Can you work these out from the model? Positions are in its coordinate system, mm. A direction names the side the tool comes from. Give positions to 0.01 mm unless a question says otherwise; leave off trailing zeros. Write each loop counter-clockwise with the first axis right and the second up, starting at its lowest first coordinate (ties: lowest second). Pieces come first, ordered by that corner, then holes. Notation, with made-up numbers: (-5, 43.5) - (39, 43.5) arc R13 ccw to (39, 52.5) - close; hole circle Ø8 at (89.25, -35.75). An arc over 180 degrees is marked (long way). Return JSON: item names as keys, results as strings. Group by question number.
from build123d import *

# Parameters (mm, degrees)
F2_R     = 10.5023561171
F3_DEPTH = 2.032
F4_R     = 1.2264204897
F6_R     = 8.280415088
F6_R_2   = 5.5395009723
F7_DEPTH = 5.334


# Not quite as in the source:
# - a fillet or chamfer that OpenCascade refuses, or shapes differently, is made with other operations: its cross-section is extruded or revolved along the edge and cut away or added


with BuildPart() as f1:
    # F0 (on Front) → F1 (revolve)
    with BuildSketch(Plane.XZ):
        with BuildLine():
            Line((0, 24.7002821416), (0, 0))
            Line((0, 0), (12.7, 0))
            ThreePointArc((12.7, 0), (15.1592770153, 1.3591062743), (12.7, 2.7182125486))
            ThreePointArc((12.7, 2.7182125486), (8.1323573281, 11.5574154189), (6.618256215, 21.3911514729))
            ThreePointArc((6.618256215, 21.3911514729), (7.1000680202, 23.0457168072), (6.618256215, 24.7002821416))
            Line((6.618256215, 24.7002821416), (0, 24.7002821416))
        make_face()
    revolve(axis=Axis((0, 0, 12.3501410708), (0, 0, -1)))

    # F2 (on face) → F3 (join)
    with BuildSketch(Plane.XY.offset(24.7002821416)):
        Circle(F2_R)
    extrude(amount=F3_DEPTH)

    # F4
    f4_edges = [f1.edges().sort_by_distance(p)[0] for p in [
        (-10.502356, 0, 26.732282),
    ]]
    fillet(f4_edges, radius=F4_R)

    # F5: fillet of radius 5.5188922036 on 1 edges, made by hand

    # F5_s1 → F5_t2 (revolve, cut)
    with BuildSketch(Plane.XZ):
        with BuildLine():
            ThreePointArc((10.5023561171, 25.5058616519), (9.1222760715, 24.9054922023), (7.631318916, 24.7002821416))
            Line((7.631318916, 24.7002821416), (7.631318916, 24.5899042975))
            Line((7.631318916, 24.5899042975), (10.5023561171, 24.5899042975))
            Line((10.5023561171, 24.5899042975), (10.6127339612, 24.7002821416))
            ThreePointArc((10.6127339612, 24.7002821416), (10.6127339612, 25.1030718967), (10.5597768612, 25.411595398))
            Line((10.5597768612, 25.411595398), (10.5023561171, 25.5058616519))
        make_face()
    revolve(axis=Axis((0, 0, 24.7002821416), (0, 0, 1)), mode=Mode.SUBTRACT)

    # F6 (on face) → F7 (join)
    with BuildSketch(Plane.XY.offset(26.7322821416)):
        Circle(F6_R)
        Circle(F6_R_2, mode=Mode.SUBTRACT)
    extrude(amount=F7_DEPTH)


solid = f1.part
1) Will these pins go through, and if not, where does the flat tip stop? pin 1 Ø8 at (x, y) = (11.5, 10.5) entering from +Z; pin 2 Ø1.5 at (x, y) = (0.5, -1) entering from +Z; pin 3 Ø3 at (y, z) = (-1.5, 22.5) entering from +X; pin 4 Ø1 at (x, z) = (-8.5, 13.5) entering from +Y.
2) I need wall thicknesses on line 1 along Y through (x, z) = (0, 30.35); line 2 along Z through (x, y) = (-1, 6.5); line 3 along Z through (x, y) = (-7.5, 6). Which ranges of each line are inside material? Lowest first, please.
3) Imagine slicing it at B-B, the plane z = 28.5. Write out the boundary of the cut face in (x, y).
4) Imagine slicing it at D-D, the plane z = 10.5. Write out the boundary of the cut face in (x, y), and give its area (3 significant figures).
5) Imagine slicing it at A-A, the plane x = 0. Write out the boundary of the cut face in (y, z), and give its area (3 significant figures).
6) We'd pull the mould along Y, two halves only. Please class faces 4 (the face through (0, 0, 26.732)), 5 (the face through (-2, -5.4, 32.066)), 6 (the face through (-6.6, -5, 29.4)): pulls with the +Y half, pulls with the -Y half, needs draft (parallel to the pull), parting line crosses it, or undercut.
7) On a 3-axis mill with a long thin cutter (end or side, diameter ignored), from which of +Z, -Z, +X, -X, +Y, -Y can I reach the whole of each face in a straight line? I mean faces 1 (the face through (0, 7, 24.7)), 2 (the face through (0, 0, 0)), 3 (the face through (-0.721, 5.492, 29.362)). Say none if no direction works.
Resolved:
{
 "1": {"pin 1": "z = 4.34", "pin 2": "z = 26.73", "pin 3": "x = 7.1", "pin 4": "through"},
 "2": {"line 1": "-8.28 to -5.54, 5.54 to 8.28", "line 2": "0 to 32.07", "line 3": "0 to 7.86, 25.07 to 26.69"},
 "3": {"outline": "circle Ø16.56 at (0, 0); hole circle Ø11.08 at (0, 0)"},
 "4": {"outline": "circle Ø17 at (0, 0)", "area": "227 mm^2"},
 "5": {"outline": "(-12.7, 0) - (12.7, 0) arc R1.61 ccw (long way) to (12.7, 2.72) arc R30.83 cw to (6.62, 21.39) arc R3.08 ccw to (6.62, 24.7) - (7.63, 24.7) arc R5.52 ccw to (10.5, 25.51) arc R1.23 ccw to (9.28, 26.73) - (8.28, 26.73) - (8.28, 32.07) - (5.54, 32.07) - (5.54, 26.73) - (-5.54, 26.73) - (-5.54, 32.07) - (-8.28, 32.07) - (-8.28, 26.73) - (-9.28, 26.73) arc R1.23 ccw to (-10.5, 25.51) arc R5.52 ccw to (-7.63, 24.7) - (-6.62, 24.7) arc R3.08 ccw to (-6.62, 21.39) arc R30.83 cw to (-12.7, 2.72) arc R1.61 ccw (long way) to start", "area": "517 mm^2"},
 "6": {"face 4": "undercut", "face 5": "needs draft", "face 6": "parting line crosses it"},
 "7": {"face 1": "none", "face 2": "-Z", "face 3": "+Z"}
}
